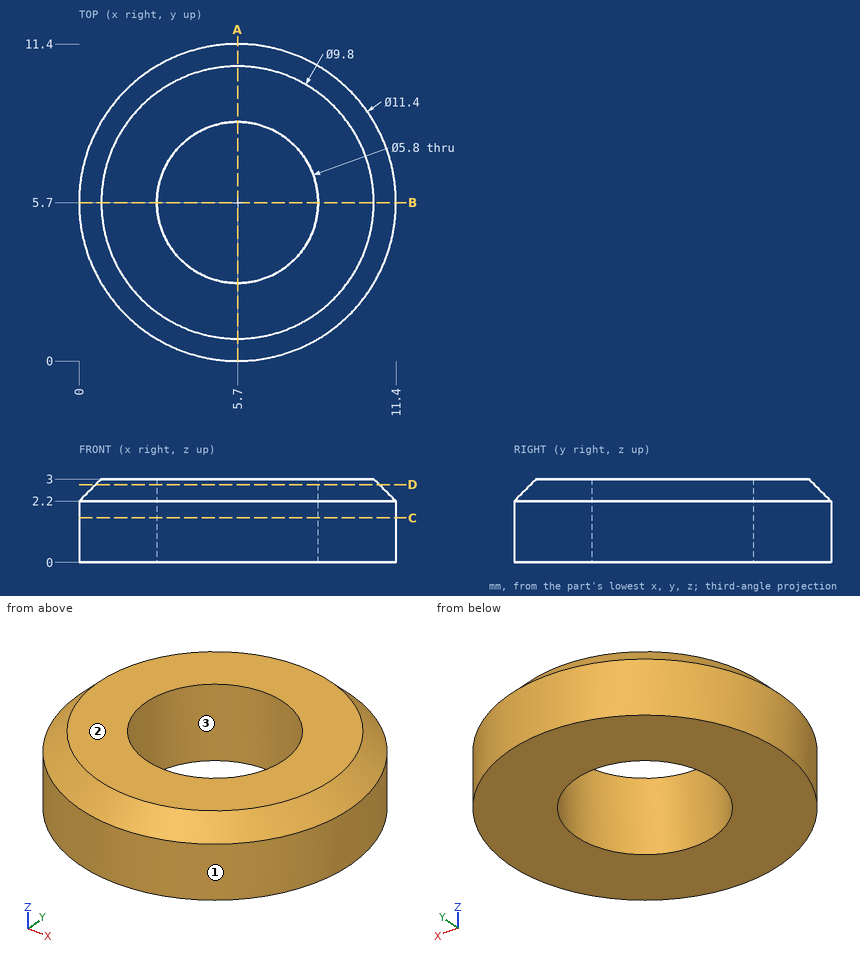
Part print with two shaded views. Sizes in mm from the minimum x, y, z corner. Round coordinates to 2 decimals unless told otherwise and drop trailing zeros. Write each loop counter-clockwise with the first axis right and the second up, starting at its lowest first coordinate (ties: lowest second). Pieces come first, ordered by that corner, then holes. Notation, with made-up numbers: M 28,46 L 86,46 A22 ccw 86,69 Z; hole C 52,26 d6. An arc over 180 degrees is marked long. Use CSV: the item, a comma, the result in double quotes.
1. Wall check: probe 1 along Y at (x, z) = (5.7, 0.9); probe 2 along X at (y, z) = (4.75, 0.4); probe 3 along X at (y, z) = (3.5, 2.4). Give the ranges that are in metal, low to high. Write a range as from..to.
Reply:
probe 1,"y = 0..2.8, 8.6..11.4"
probe 2,"x = 0.08..2.96, 8.44..11.32"
probe 3,"x = 0.66..3.81, 7.59..10.74"
2. Saw through at C-C (z = 1.6). Give the cut face in (x, y), plus the area to 3 significant figures.
Reply:
outline,"C 5.7,5.7 d11.4; hole C 5.7,5.7 d5.8"
area,"75.6 mm²"
3. Saw through at A-A (x = 5.7). Give the cut face in (y, z), plus the area to 3 significant figures.
Reply:
outline,"M 0,0 L 2.8,0 L 2.8,3 L 0.8,3 L 0,2.2 Z; M 8.6,0 L 11.4,0 L 11.4,2.2 L 10.6,3 L 8.6,3 Z"
area,"16.2 mm²"
4. Two-plate mould, pull along Y, no slides. Class the marked faces 1, 2 and 3: +Y half, -Y half, draft (parallel to the pull), parting line (faces both ways), or undercut.
Reply:
face 1,"parting line"
face 2,"draft"
face 3,"undercut"
5. Saw through at D-D (z = 2.8). Give the cut face in (x, y).
Reply:
outline,"C 5.7,5.7 d10.2; hole C 5.7,5.7 d5.8"
6. Flat gauge pins, fed straight in: pin 1 (1.5 mm diameter, centred on x = 1.5, z = 1.5, fed in from +Y); pin 2 (4.5 mm diameter, centred on x = 5.7, y = 5.7, fed in from -Z); pin 3 (1 mm diameter, centred on x = 1, z = 0.5, fed in from +Y); pin 4 (1.5 mm diameter, centred on y = 1.5, z = 1, fed in from +X). Where does each tip first touch, or does it go through?
Reply:
pin 1,"stops at y = 10.24"
pin 2,"passes through"
pin 3,"stops at y = 9.55"
pin 4,"stops at x = 10.24"
